The figure shows three views and two pictorial views of one solid part (mm, origin at its lowest corner). Answer the questions. A direction names the side the tool comes from. Round coordinates to 2 decimals unless told otherwise and drop trailing zeros. Write each loop counter-clockwise with the first axis right and the second up, starting at its lowest first coordinate (ties: lowest second). Pieces come first, ordered by that corner, then holes. Notation, with made-up numbers: (44.5, 3.25) - (92.5, 3.25) arc R34 ccw to (92.5, 38.25) - close; hole circle Ø5 at (82.5, 48). An arc over 180 degrees is marked (long way). Answer as CSV lines item,"result". Start each with the question number.
Item 1: Flat-ended cylindrical pins translate along their axes: pin 1 (1.3 mm diameter, centred on x = 17, z = 1, fed in from -Y) (1 decimal); pin 2 (2.5 mm diameter, centred on x = 1.5, z = 3.5, fed in from +Y); pin 3 (1 mm diameter, centred on x = 15.5, z = 4, fed in from +Y). Find the tip coordinate at first contact, or state that the pin passes through.
Item 2: A cutting plane is placed at C-C on y = 12.7. Determine the outline of the cut face in (x, z).
Item 3: A cutting plane is placed at A-A on x = 39.37. State how many separate pieces and enclosed holes the cut face has.
Item 4: A cutting plane is placed at B-B on x = 11.43. Determine the outline of the cut face in (y, z).
Item 5: Straight lines are drawn through the part: line 1 along X through (y, z) = (12.7, 0.9); line 2 along X through (y, z) = (2, 8.5); line 3 along Z through (x, y) = (28.5, 9.5). For each, find the intervals that lie inside material, in ascending order. Write a range as [from, to].
Item 6: Which of the six approach directions +Z, -Z, +X, -X, +Y, -Y give full straight-line access (tool end or side, diameter ignored) to the marked faces 4 and 5?
Item 7: For a pull along X with two mould halves and no side action, classify the marked faces 1, 2 and 3 as pulls with the +X half, pulls with the -X half, needs draft (parallel to the pull), parting line crosses it, or undercut.
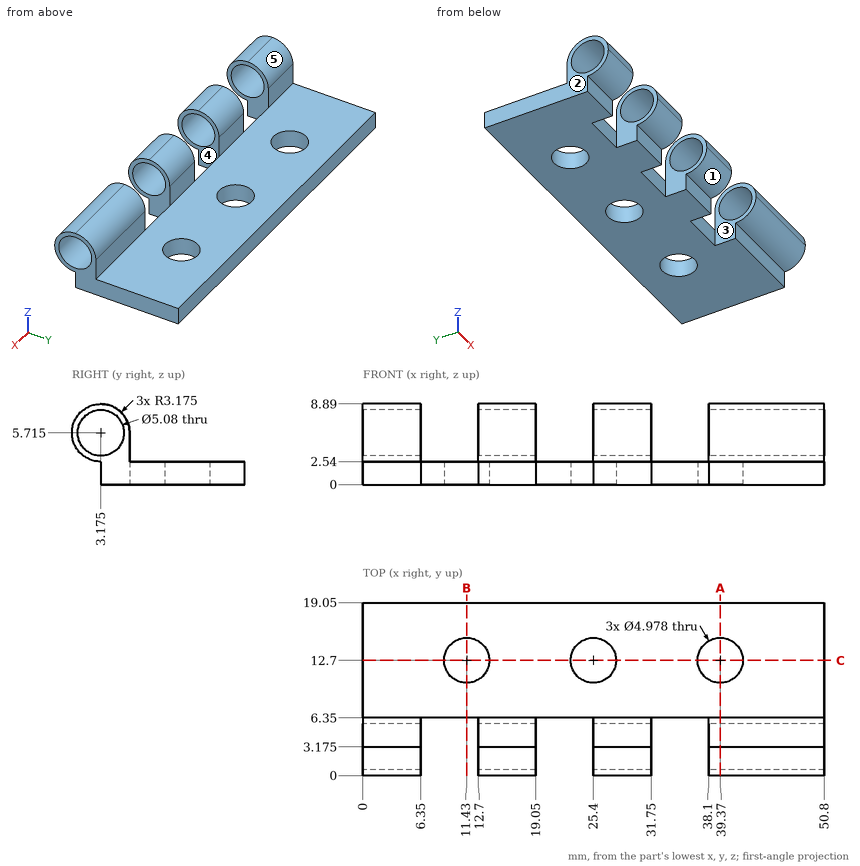
Geometry says:
1,pin 1,"stops at y = 3.2"
1,pin 2,"stops at y = 19.05"
1,pin 3,"stops at y = 6.35"
2,outline,"(0, 0) - (8.94, 0) - (8.94, 2.54) - (0, 2.54) - close; (13.92, 0) - (22.91, 0) - (22.91, 2.54) - (13.92, 2.54) - close; (27.89, 0) - (36.88, 0) - (36.88, 2.54) - (27.89, 2.54) - close; (41.86, 0) - (50.8, 0) - (50.8, 2.54) - (41.86, 2.54) - close"
3,separate pieces,"2"
3,enclosed holes,"1"
4,outline,"(6.35, 0) - (10.21, 0) - (10.21, 2.54) - (6.35, 2.54) - close; (15.19, 0) - (19.05, 0) - (19.05, 2.54) - (15.19, 2.54) - close"
5,line 1,"x = [0, 8.94], [13.92, 22.91], [27.89, 36.88], [41.86, 50.8]"
5,line 2,"x = [0, 6.35], [12.7, 19.05], [25.4, 31.75], [38.1, 50.8]"
5,line 3,"z = [0, 2.54]"
6,face 4,"+Z, -Z, -Y"
6,face 5,"+Z, +X, -X, +Y"
7,face 1,"needs draft"
7,face 2,"pulls with the -X half"
7,face 3,"undercut"
